For this review, take the finished solid that the model builds, in its own axes (mm). A direction names the side the tool comes from. Give positions to 0.01 mm unless a question says otherwise; leave off trailing zeros. Order: outer loops, then holes, each group sorted by start corner. A loop starts at its lowest first (then second) coordinate and runs counter-clockwise, first axis right, second up. Notation, with made-up numbers: (9.5, 46.25) - (22.5, 46.25) arc R20 cw to (22.5, 80.25) - close; hole circle Ø7 at (-31.75, 54). An arc over 180 degrees is marked (long way). Use a Markdown table: item, result. Add a question column.
1) Clearance check with flat-ended pins moving along their axes: P1, Ø4, axis at x = -4, y = -4.5, coming from the +Z side; P2, Ø1, axis at x = -2.5, z = 1, coming from the -Y side; P3, Ø1.5, axis at x = -4.5, z = 2, coming from the +Y side. State where each tip first meets the part, or that it passes through.
2) Mouldability with a two-part tool opening along Y and no side actions: class faces 1 (the face through (3, -1, 0)), 2 (the face through (-0.338, 2.578, 2.021)), 3 (the face through (-4.385, 4.021, 0.74)) as released by +Y, released by -Y, zero draft, split by the parting line, or undercut.
3) We need section D-D on z = 3.15. Write out the cut boundary in (x, y).
4) Wall thickness on L1, parallel to Y at x = 0, z = 2.65; L2, parallel to Z at x = -3, y = -3.25; L3, parallel to Y at x = 0, z = 1.8: over which ranges is each line inside the solid? List them lowest first.
5) Machinability: for faces 4 (the face through (0, 3, 4.1)), 5 (the face through (-4, 3, 1.5)), which of the approach directions +Z, -Z, +X, -X, +Y, -Y give a long, thin tool a straight path to every point of the face, cutting with its end or side? Answer none if there is none.
6) We need section A-A on x = 0. Write out the cut boundary in (y, z).
7) We need section C-C on z = 0.95. Write out the cut boundary in (x, y).
```python
from build123d import *

# Parameters (mm, degrees)
SKETCH_1_R          = 5.95
SKETCH_1_R_2        = 3.5
EXTRUDE_1_DEPTH     = 1.5
SKETCH_1_2_R        = 3.5
EXTRUDE_2_DEPTH     = 4.1
SKETCH_2_R          = 2.6
CUT_EXTRUDE_1_DEPTH = 10.360288457
FILLET_1_R          = 1


with BuildPart() as part:
    # 草图1 → 凸台-拉伸1 (new body)
    with BuildSketch(Plane.XY):
        Circle(SKETCH_1_R)
        Circle(SKETCH_1_R_2, mode=Mode.SUBTRACT)
    extrude(amount=EXTRUDE_1_DEPTH)

    # 草图1<2> → 凸台-拉伸2 (add)
    with BuildSketch(Plane.XY):
        Circle(SKETCH_1_2_R)
    extrude(amount=EXTRUDE_2_DEPTH)

    # 草图2 → 切除-拉伸1 (cut, through all)
    with BuildSketch(Plane.XY):
        Circle(SKETCH_2_R)
    extrude(amount=CUT_EXTRUDE_1_DEPTH, mode=Mode.SUBTRACT)

    # 圆角1
    fillet_1_edges = [part.edges().sort_by_distance(p)[0] for p in [
        (-3.5, 0, 1.5),
    ]]
    fillet(fillet_1_edges, radius=FILLET_1_R)


solid = part.part
```
Checked values:
| question | item | result |
|---|---|---|
| 1 | P1 | z = 1.62 |
| 1 | P2 | y = -5.6 |
| 1 | P3 | y = 4.46 |
| 2 | face 1 | zero draft |
| 2 | face 2 | undercut |
| 2 | face 3 | split by the parting line |
| 3 | outline | circle Ø7 at (0, 0); hole circle Ø5.2 at (0, 0) |
| 4 | L1 | -3.5 to -2.6, 2.6 to 3.5 |
| 4 | L2 | 0 to 1.5 |
| 4 | L3 | -3.79 to -2.6, 2.6 to 3.79 |
| 5 | face 4 | +Z, +X, -X, +Y, -Y |
| 5 | face 5 | +Z |
| 6 | outline | (-5.95, 0) - (-2.6, 0) - (-2.6, 4.1) - (-3.5, 4.1) - (-3.5, 2.5) arc R1 cw to (-4.5, 1.5) - (-5.95, 1.5) - close; (2.6, 0) - (5.95, 0) - (5.95, 1.5) - (4.5, 1.5) arc R1 cw to (3.5, 2.5) - (3.5, 4.1) - (2.6, 4.1) - close |
| 7 | outline | circle Ø11.9 at (0, 0); hole circle Ø5.2 at (0, 0) |
